Design review of the part shown in the three views and the two pictorial views. Dimensions are in mm from the part's minimum x, y and z. A direction names the side the tool comes from. Give positions to 0.01 mm unless a question says otherwise; leave off trailing zeros. Write each loop counter-clockwise with the first axis right and the second up, starting at its lowest first coordinate (ties: lowest second). Pieces come first, ordered by that corner, then holes. Notation, with made-up numbers: M 14.5,-5 L 48.5,-5 A8 ccw 48.5,7 Z; hole C -20.75,-15 d3. An arc over 180 degrees is marked long. Write item = value, one per line.
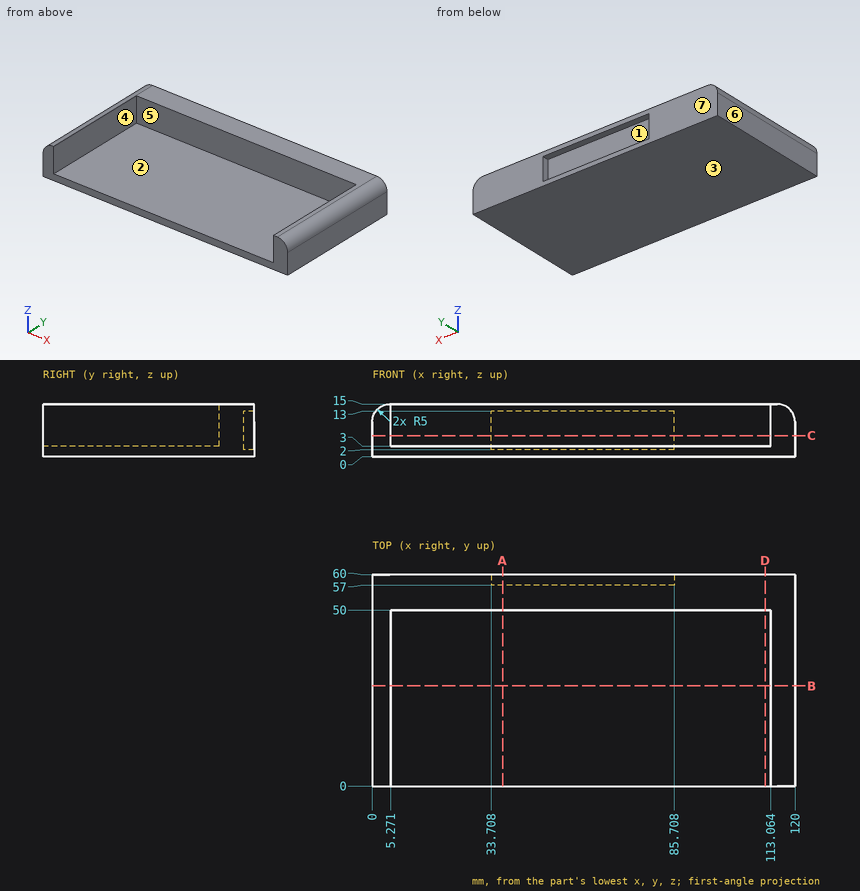
1. The part is to be moulded in two halves that separate along X. For the marked faces 4, 5, 6 and 7, say which applies: +X half, -X half, draft (parallel to the pull), parting line (faces both ways), or undercut.
Responses:
face_4 = undercut
face_5 = undercut
face_6 = -X half
face_7 = draft
2. We need section A-A, the plane x = 37. Write out the cut boundary in (y, z), then the cut area to 3 significant figures.
Responses:
outline = M 0,0 L 60,0 L 60,2 L 57,2 L 57,13 L 60,13 L 60,15 L 50,15 L 50,3 L 0,3 Z
area = 267 mm2
3. We need section D-D, the plane x = 111.5. Write out the cut boundary in (y, z).
Responses:
outline = M 0,0 L 60,0 L 60,15 L 50,15 L 50,3 L 0,3 Z
4. Insertion check: P1, Ø3.5, axis at x = 53.5, z = 9.5, coming from the +Y side; P2, Ø6, axis at x = 94, y = 16, coming from the +Z side; P3, Ø1, axis at x = 34.5, z = 10, coming from the -Y side. Each pin has a flat end and moves straight along its axis. Give the tip position at first contact, or say it passes through.
Responses:
P1 = 57
P2 = 3
P3 = 50
5. For line 1 along X through (y, z) = (38, 10.5) (1 decimal); line 2 along Y through (x, z) = (53, 9.5); line 3 along Z through (x, y) = (77.5, 31.5), list the stretches that pass through material, from the lowest coordinate up. Write a range as from..to.
Responses:
line_1 = 0..5.3, 113.1..120
line_2 = 50..57
line_3 = 0..3
6. Machinability: for the marked faces 1, 2 and 3, which of the approach directions +Z, -Z, +X, -X, +Y, -Y give a long, thin tool a straight path to every point of the face, cutting with its end or side? Answer none if there is none.
Responses:
face_1 = +Y
face_2 = +Z, -Y
face_3 = -Z, +X, -X, +Y, -Y
7. We need section C-C, the plane z = 6. Write out the cut boundary in (x, y), then the cut area to 3 significant figures.
Responses:
outline = M 0,0 L 5.27,0 L 5.27,50 L 113.06,50 L 113.06,0 L 120,0 L 120,60 L 85.71,60 L 85.71,57 L 33.71,57 L 33.71,60 L 0,60 Z
area = 1,650 mm2
8. We need section B-B, the plane y = 28.5. Write out the cut boundary in (x, z).
Responses:
outline = M 0,0 L 120,0 L 120,10 A5 ccw 115,15 L 113.06,15 L 113.06,3 L 5.27,3 L 5.27,15 L 5,15 A5 ccw 0,10 Z
